from build123d import *

# Parameters (mm, degrees)
F0_R          = 6.096
F1_DEPTH      = 25.4
F2_R          = 4.318
F3_R          = 0.79375
F4_DEPTH      = 6.097
F4_DEPTH_BACK = 6.097
F6_DEPTH      = 6.0970001
F6_DEPTH_BACK = 6.0970001
F7_R          = 0.2032


with BuildPart() as f1:
    # F0 (on Top) → F1 (new body)
    with BuildSketch(Plane.XY):
        Circle(F0_R)
    extrude(amount=F1_DEPTH)

    # F2
    f2_edges = [f1.edges().sort_by_distance(p)[0] for p in [
        (-6.096, 0, 25.4),
    ]]
    fillet(f2_edges, radius=F2_R)

    # F3 (on Front) → F4 (cut, two sides)
    with BuildSketch(Plane.XZ) as f4_sk:
        with Locations((0, 2.54)):
            Circle(F3_R)
    extrude(amount=-F4_DEPTH, mode=Mode.SUBTRACT)
    extrude(f4_sk.sketch, amount=F4_DEPTH_BACK, mode=Mode.SUBTRACT)

    # F5 (on Right) → F6 (cut, two sides)
    with BuildSketch(Plane.YZ) as f6_sk:
        with BuildLine():
            Line((-3.81, 0), (0, 0))
            Line((0, 0), (3.81, 0))
            Line((3.81, 0), (3.81, 4.572))
            ThreePointArc((3.81, 4.572), (0, 8.382), (-3.81, 4.572))
            Line((-3.81, 4.572), (-3.81, 0))
        make_face()
    extrude(amount=-F6_DEPTH, mode=Mode.SUBTRACT)
    extrude(f6_sk.sketch, amount=F6_DEPTH_BACK, mode=Mode.SUBTRACT)

    # F7
    f7_edges = [f1.edges().sort_by_distance(p)[0] for p in [
        (-4.758688, -3.81, 2.286),
        (4.758688, -3.81, 2.286),
        (5.465335, 2.700246, 7.259894),
        (-6.096, 0, 8.382),
        (5.465335, -2.700246, 7.259894),
        (4.758688, 3.81, 2.286),
        (-4.758688, 3.81, 2.286),
    ]]
    fillet(f7_edges, radius=F7_R)


solid = f1.part
Work out the finished part from the listing and answer in its coordinate system (mm). A direction names the side the tool comes from. Round coordinates to 2 decimals unless told otherwise and drop trailing zeros. Loops run counter-clockwise (first coordinate to the right, second up) from the corner with the lowest first, then second, coordinate; pieces in that order, holes last. Notation, with made-up numbers: M 86,57.25 L 130,57.25 A19 ccw 130,89.25 Z; hole C -19,6 d5. An arc over 180 degrees is marked long. One line per question, with ' | ' between items. Start each with the question number.
(1) A cutting plane is placed at A-A on z = 2.25. Write down the section's boundary in (x, y).
(2) A cutting plane is placed at C-C on z = 13.5. Write down the section's boundary in (x, y), plus the area to 3 significant figures.
(3) A cutting plane is placed at B-B on x = 0. Give the number of separate pieces and of enclosed holes in the cut face, plus the area to 3 significant figures.
(4) A tool of negligible diameter and unlimited length cuts with its end or side. For faces 4 (the face through (5.814, 1.831, 12.736)), 5 (the face through (-1, 3.81, 2)), from which of +Z, -Z, +X, -X, +Y, -Y can it reach the whole face along a straight path? Write none if from no direction.
(5) Find the intervals of material crossed by line 1 (X direction, y = 4.8, z = 2.54); line 2 (Z direction, x = 0, y = 5.55); line 3 (X direction, y = 4.7, z = 2.54), in increasing order.
(6) For a pull along Z with two mould halves and no side action, classify faces 1 (the face through (-0.103, 4.937, 3.327)), 2 (the face through (1, -3.81, 2)), 3 (the face through (-0.08, 0.08, 8.38)) as released by +Z, released by -Z, zero draft, split by the parting line, or undercut.
(7) Flat-ended cylindrical pins translate along their axes: pin 1 Ø6 at (x, y) = (0, -3) entering from -Z; pin 2 Ø6 at (y, z) = (-3.5, 8.5) entering from +X; pin 3 Ø4 at (x, z) = (2.5, 20.5) entering from -Y; pin 4 Ø1 at (x, z) = (-3, 7) entering from +Y. Find the tip coordinate at first contact, or state that the pin passes through.
Geometry check:
1) outline: M -4.46,-4.15 A6.1 ccw -0.74,-6.05 L -0.74,-3.81 L -4.32,-3.81 A0.2 ccw Z; M -4.46,4.15 A0.2 ccw -4.32,3.81 L -0.74,3.81 L -0.74,6.05 A6.1 ccw Z; M 0.74,-6.05 A6.1 ccw 4.46,-4.15 A0.2 ccw 4.32,-3.81 L 0.74,-3.81 Z; M 0.74,3.81 L 4.32,3.81 A0.2 ccw 4.46,4.15 A6.1 ccw 0.74,6.05 Z
2) outline: C 0,0 d12.19 | area: 117 mm²
3) separate pieces: 3 | enclosed holes: 0 | area: 237 mm²
4) face 4: +Z, -Z | face 5: -Z, +X, -X
5) line 1: x = -3.76 to -0.79, 0.79 to 3.76 | line 2: z = 0 to 1.75, 3.33 to 23.18 | line 3: x = -3.88 to -0.79, 0.79 to 3.88
6) face 1: undercut | face 2: zero draft | face 3: released by -Z
7) pin 1: stops at z = 0 | pin 2: stops at x = 6.08 | pin 3: stops at y = -6.08 | pin 4: stops at y = 5.56
